```python
from build123d import *

# Parameters (mm, degrees)
F0_R      = 17.78
F1_DEPTH  = 2.54
F2_R      = 17.78
F2_R_2    = 16.51
F3_DEPTH  = 1.27
F4_R      = 17.78
F5_DEPTH  = 2.54
F6_R      = 14.605
F7_DEPTH  = 50.8
F8_R      = 2.54
F10_DEPTH = 30.734


with BuildPart() as f1:
    # F0 (on Top) → F1 (new body)
    with BuildSketch(Plane.XY):
        Circle(F0_R)
    extrude(amount=F1_DEPTH)

    # F2 (on face) → F3 (join)
    with BuildSketch(Plane.XY.offset(2.54)):
        Circle(F2_R)
        Circle(F2_R_2, mode=Mode.SUBTRACT)
    extrude(amount=F3_DEPTH)

    # F4 (on face) → F5 (join)
    with BuildSketch(Plane.XY.offset(3.81)):
        Circle(F4_R)
    extrude(amount=F5_DEPTH)

    # F6 (on face) → F7 (cut)
    with BuildSketch(Plane(origin=(0, 0, 0), x_dir=(1, 0, 0), z_dir=(0, 0, -1))):
        Circle(F6_R)
    extrude(amount=-F7_DEPTH, mode=Mode.SUBTRACT)

    # F8
    f8_edges = [f1.edges().sort_by_distance(p)[0] for p in [
        (-17.78, 0, 6.35),
        (-17.78, 0, 0),
    ]]
    fillet(f8_edges, radius=F8_R)

    # F9 (on face) → F10 (cut)
    with BuildSketch(Plane.XY.offset(6.35)):
        with BuildLine():
            Line((-3.4012887627, -22.1683233976), (3.4012887627, -22.1683233976))
            Line((3.4012887627, -22.1683233976), (3.4012887627, -14.855599441))
            ThreePointArc((3.4012887627, -14.855599441), (0, -15.24), (-3.4012887627, -14.855599441))
            Line((-3.4012887627, -14.855599441), (-3.4012887627, -22.1683233976))
        make_face()
        with BuildLine():
            ThreePointArc((-3.4012887627, -14.2034242263), (0, -14.605), (3.4012887627, -14.2034242263))
            Line((3.4012887627, -14.2034242263), (3.4012887627, -10.824047029))
            Line((3.4012887627, -10.824047029), (-3.4012887627, -10.824047029))
            Line((-3.4012887627, -10.824047029), (-3.4012887627, -14.2034242263))
        make_face()
        with BuildLine():
            ThreePointArc((-3.4012887627, -14.855599441), (0, -15.24), (3.4012887627, -14.855599441))
            Line((3.4012887627, -14.855599441), (3.4012887627, -14.2034242263))
            ThreePointArc((3.4012887627, -14.2034242263), (0, -14.605), (-3.4012887627, -14.2034242263))
            Line((-3.4012887627, -14.2034242263), (-3.4012887627, -14.855599441))
        make_face()
    extrude(amount=-F10_DEPTH, mode=Mode.SUBTRACT)


solid = f1.part
```
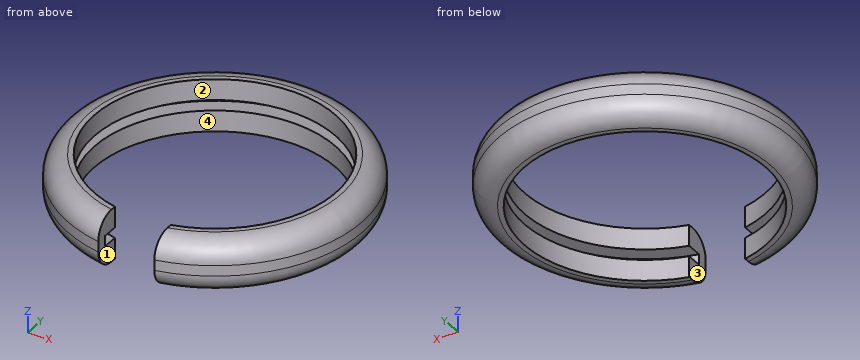
Can you work these out from the model? Positions are in its coordinate system, mm. Face numbers are marked on the shaded views. A direction names the side the tool comes from. Give positions to 0.01 mm unless a question says otherwise; leave off trailing zeros. Loops run counter-clockwise (first coordinate to the right, second up) from the corner with the lowest first, then second, coordinate; pieces in that order, holes last. Notation, with made-up numbers: M -13,70.25 L 16,70.25 A25 cw 16,105.25 Z; hole C 66,65.25 d7. An arc over 180 degrees is marked long. One line per question, with ' | ' between items. Start each with the question number.
Q1. For pin 1 Ø2 at (y, z) = (7, 1) entering from +X; pin 2 Ø1.6 at (y, z) = (-16, 3) entering from +X; pin 3 Ø1.6 at (y, z) = (-16.5, 2.5) entering from -X, each with a flat end and sliding along its axis, tell me the tip position at first contact or that it passes through.
Q2. If we section it at A-A (y = 0): Please give me the cut outline in (x, z) (3 decimals), plus the area to 3 significant figures.
Q3. For the marked faces 3 and 4, which set-ups out of +Z, -Z, +X, -X, +Y, -Y let a thin tool reach every point of the face, with its end or its side?
Q4. If we section it at B-B (x = 0): Please give me the cut outline in (y, z) (3 decimals), plus the area to 3 significant figures.
Q5. If we section it at C-C (z = 3): Please give me the cut outline in (x, y).
Q6. If we mould it in two halves opening along Y, with no side actions, what happens to the marked faces 1 and 2? For each: +Y half, -Y half, draft (parallel to the pull), parting line (faces both ways), or undercut.
Q7. If we section it at D-D (z = 5.25): Please give me the cut outline in (x, y) (3 decimals), plus the area to 3 significant figures.
Q8. If I drill on line 1 (Z direction, x = 14.5, y = 5); line 2 (Y direction, x = 6, z = 0.75); line 3 (X direction, y = 1.5, z = 2), over which ranges is the centre line in solid material (lowest first)? Write a range as from..to.
Computed:
1) pin 1: stops at x = 16.48 | pin 2: stops at x = 9.22 | pin 3: stops at x = -8.34
2) outline: M -17.78,2.54 A2.54 ccw -15.24,0 L -14.605,0 L -14.605,2.54 L -16.51,2.54 L -16.51,3.81 L -14.605,3.81 L -14.605,6.35 L -15.24,6.35 A2.54 ccw -17.78,3.81 Z; M 14.605,0 L 15.24,0 A2.54 ccw 17.78,2.54 L 17.78,3.81 A2.54 ccw 15.24,6.35 L 14.605,6.35 L 14.605,3.81 L 16.51,3.81 L 16.51,2.54 L 14.605,2.54 Z | area: 29.9 mm²
3) face 3: +Z, -Z, -Y | face 4: +Z, -Z
4) outline: M 14.605,0 L 15.24,0 A2.54 ccw 17.78,2.54 L 17.78,3.81 A2.54 ccw 15.24,6.35 L 14.605,6.35 L 14.605,3.81 L 16.51,3.81 L 16.51,2.54 L 14.605,2.54 Z | area: 15.0 mm²
5) outline: M -3.4,-17.45 L -3.4,-16.16 A16.51 cw long 3.4,-16.16 L 3.4,-17.45 A17.78 ccw long Z
6) face 1: draft | face 2: undercut
7) outline: M -3.401,-16.995 L -3.401,-14.203 A14.605 cw long 3.401,-14.203 L 3.401,-16.995 A17.332 ccw long Z | area: 255 mm²
8) line 1: z = 0..2.54, 3.81..6.35 | line 2: y = -15.95..-13.32, 13.32..15.95 | line 3: x = -17.66..-14.53, 14.53..17.66
